Geometry check sheet. Reference: drawing and pictorial views, mm from the part's lowest x, y, z. Give positions to 0.01 mm unless a question says otherwise; leave off trailing zeros. Write each loop counter-clockwise with the first axis right and the second up, starting at its lowest first coordinate (ties: lowest second). Pieces come first, ordered by that corner, then holes. Notation, with made-up numbers: (76.5, -22) -> (116.5, -22) arc R13 cw to (116.5, -1) -> close; hole circle Ø8 at (65.25, -6.75). An arc over 180 degrees is marked (long way). Return JSON: item names as keys, results as strings.
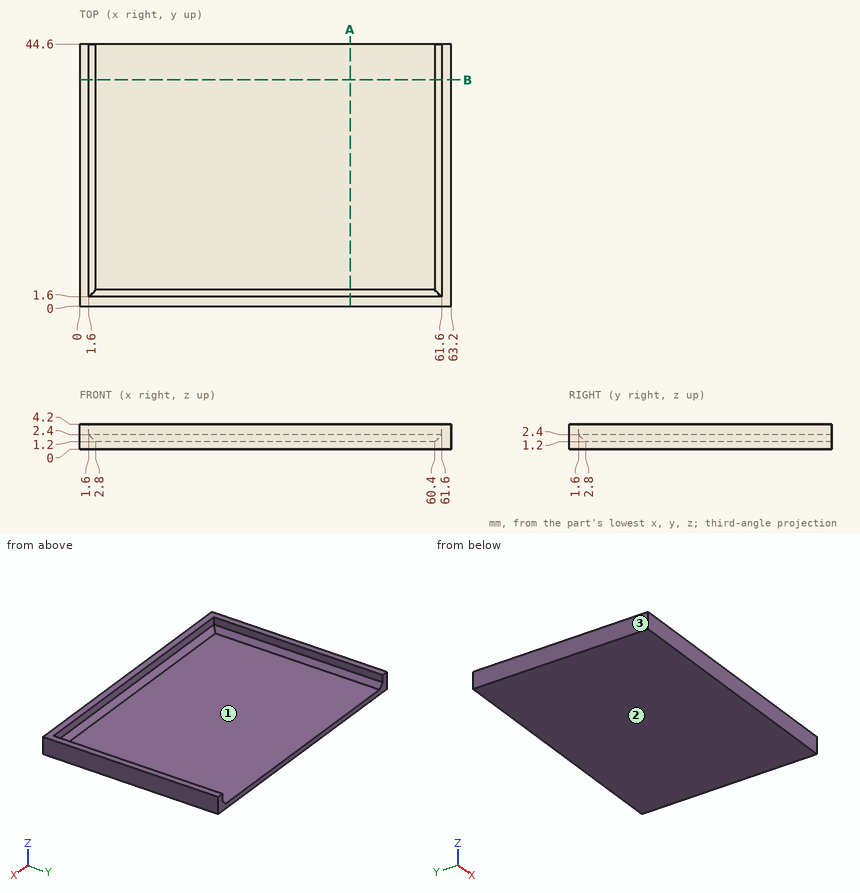
(1) Release check for a two-part mould opening along X. For the marked faces 1, 2 and 3 record: pulls with the +X half, pulls with the -X half, needs draft (parallel to the pull), parting line crosses it, or undercut.
Reply:
{"face 1": "undercut", "face 2": "needs draft", "face 3": "pulls with the -X half"}
(2) Cross-section at B-B on y = 38.5. Enter the section's corners in (x, z), then the cut area to 3 significant figures.
Reply:
{"outline": "(0, 0) -> (63.2, 0) -> (63.2, 4.2) -> (61.6, 4.2) -> (61.6, 2.4) -> (60.4, 1.2) -> (2.8, 1.2) -> (1.6, 2.4) -> (1.6, 4.2) -> (0, 4.2) -> close", "area": "86.9 mm^2"}
(3) Depth check by flat-ended pin: pin 1 Ø12.5 at (x, y) = (40, 16) entering from +Z; pin 2 Ø0.9 at (x, z) = (35.5, 3.5) entering from +Y. Enter the tip coordinate at first touch or a pass-through.
Reply:
{"pin 1": "z = 1.2", "pin 2": "y = 1.6"}
(4) Thickness scan on L1, parallel to X at y = 23, z = 2.4; L2, parallel to Z at x = 49, y = 6; L3, parallel to Y at x = 6, z = 3.55. Record the ranges inside material, lowest first.
Reply:
{"L1": "0 to 1.6, 61.6 to 63.2", "L2": "0 to 1.2", "L3": "0 to 1.6"}
(5) Cross-section at A-A on x = 46. Enter the section's corners in (y, z), then the cut area to 3 significant figures.
Reply:
{"outline": "(0, 0) -> (44.6, 0) -> (44.6, 1.2) -> (2.8, 1.2) -> (1.6, 2.4) -> (1.6, 4.2) -> (0, 4.2) -> close", "area": "59.0 mm^2"}
